Read the model definition and answer for the solid it produces. Units are mm, in the model's axes. Face numbers are marked on the shaded views. A direction names the side the tool comes from. Give positions to 0.01 mm unless a question says otherwise; leave off trailing zeros. Write each loop counter-clockwise with the first axis right and the second up, starting at its lowest first coordinate (ties: lowest second). Pieces come first, ordered by that corner, then holes. Notation, with made-up numbers: M 71.25,76 L 105.25,76 A21 ccw 105.25,80 Z; hole C 10.5,-14 d1. An arc over 180 degrees is marked long. Use a Markdown table: item, result. Add a question column.
Item 1: A cutting plane is placed at D-D on x = 6.35. Determine the outline of the cut face in (y, z).
Item 2: Given P1, Ø11, axis at x = 136.5, y = 6, coming from the -Z side (3 decimals); P2, Ø12.5, axis at x = 162.052, y = 0, coming from the -Z side; P3, Ø1, axis at y = 10, z = 7.5, coming from the -X side; P4, Ø10, axis at x = 19, z = 3.5, coming from the -Y side, each flat-ended and moving along its own axis, determine where each tip first touches the part or whether it passes through.
Item 3: A cutting plane is placed at C-C on y = 17. Determine the outline of the cut face in (x, z) (3 decimals).
Item 4: A cutting plane is placed at B-B on z = -4. Determine the outline of the cut face in (x, y) (3 decimals), then the cut area to 3 significant figures.
Item 5: For the marked faces 1, 2, 3, 4 and 5, determine the directions among +Z, -Z, +X, -X, +Y, -Y from which every point of the face is accessible in a straight line to the end or side of a thin tool.
Item 6: A cutting plane is placed at A-A on y = 0. Determine the outline of the cut face in (x, z) (3 decimals), then the cut area to 3 significant figures.
Item 7: Consider probe 1 along X at (y, z) = (0, -5.75) (3 decimals); probe 2 along X at (y, z) = (-2, -4) (3 decimals); probe 3 along X at (y, z) = (9.5, -11). Determine where each line is inside the solid, lowest interval first. Write a range as [from, to].
from build123d import *

# Parameters (mm, degrees)
F0_R          = 10.033
F1_DEPTH      = 168.275
F3_W          = 39.878
F3_H          = 74.93
F4_DEPTH      = 127
F5_W          = 39.878
F5_H          = 34.925
F6_DEPTH      = 22.225
F7_R          = 3.937
F8_DEPTH      = 19.051
F8_DEPTH_BACK = 55.881


with BuildPart() as f1:
    # F0 (on Right) → F1 (new body)
    with BuildSketch(Plane.YZ):
        Circle(F0_R)
    extrude(amount=F1_DEPTH)

    # F3 (on offset) → F4 (join)
    with BuildSketch(Plane.YZ.offset(19.05)):
        with Locations((0, -18.415)):
            Rectangle(F3_W, F3_H)
    extrude(amount=F4_DEPTH)

    # F5 (on face) → F6 (cut)
    with BuildSketch(Plane.YZ.offset(146.05)):
        with Locations((0, -38.4175)):
            Rectangle(F5_W, F5_H)
    extrude(amount=-F6_DEPTH, mode=Mode.SUBTRACT)

    # F7 (on Top) → F8 (cut, two sides)
    with BuildSketch(Plane.XY) as f8_sk:
        with Locations((6.35, 0)):
            Circle(F7_R)
        with Locations((162.052, 0)):
            Circle(F7_R)
    extrude(amount=F8_DEPTH, mode=Mode.SUBTRACT)
    extrude(f8_sk.sketch, amount=-F8_DEPTH_BACK, mode=Mode.SUBTRACT)


solid = f1.part
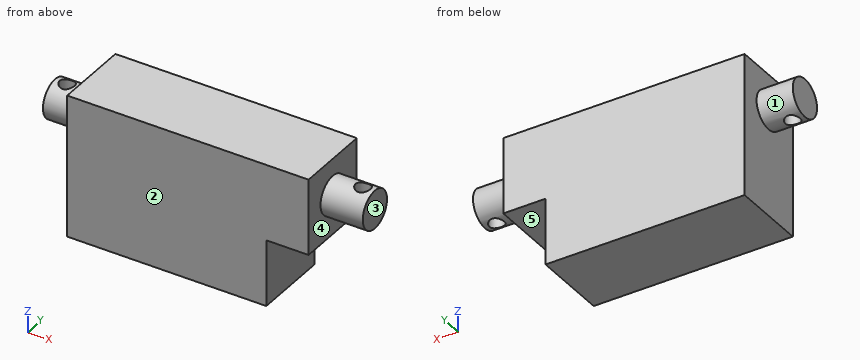
Filled in:
| question | item | result |
|---|---|---|
| 1 | outline | M -3.94,-9.23 L -3.94,9.23 A10.03 ccw Z; M 3.94,-9.23 A10.03 ccw 3.94,9.23 Z |
| 2 | P1 | z = -20.955 |
| 2 | P2 | z = -10.03 |
| 2 | P3 | x = 19.05 |
| 2 | P4 | y = -19.94 |
| 3 | outline | M 19.05,-55.88 L 123.825,-55.88 L 123.825,-20.955 L 146.05,-20.955 L 146.05,19.05 L 19.05,19.05 Z |
| 4 | outline | M 0,-9.201 L 19.05,-9.201 L 19.05,-19.939 L 146.05,-19.939 L 146.05,-9.201 L 168.275,-9.201 L 168.275,9.201 L 146.05,9.201 L 146.05,19.939 L 19.05,19.939 L 19.05,9.201 L 0,9.201 Z; hole C 6.35,0 d7.874; hole C 162.052,0 d7.874 |
| 4 | area | 5,730 mm² |
| 5 | face 1 | -X |
| 5 | face 2 | +Z, -Z, +X, -X, -Y |
| 5 | face 3 | +Z, -Z, +X, +Y, -Y |
| 5 | face 4 | +X |
| 5 | face 5 | -Z, +X, +Y, -Y |
| 6 | outline | M 0,-10.033 L 2.413,-10.033 L 2.413,10.033 L 0,10.033 Z; M 10.287,-10.033 L 19.05,-10.033 L 19.05,-55.88 L 123.825,-55.88 L 123.825,-20.955 L 146.05,-20.955 L 146.05,-10.033 L 158.115,-10.033 L 158.115,10.033 L 146.05,10.033 L 146.05,19.05 L 19.05,19.05 L 19.05,10.033 L 10.287,10.033 Z; M 165.989,-10.033 L 168.275,-10.033 L 168.275,10.033 L 165.989,10.033 Z |
| 6 | area | 9,250 mm² |
| 7 | probe 1 | [0, 2.413], [10.287, 158.115], [165.989, 168.275] |
| 7 | probe 2 | [0, 2.959], [9.741, 158.661], [165.443, 168.275] |
| 7 | probe 3 | [19.05, 146.05] |
